Geometry check sheet. Reference: drawing and pictorial views, mm from the part's lowest x, y, z. A direction names the side the tool comes from. Round coordinates to 2 decimals unless told otherwise and drop trailing zeros. Write each loop counter-clockwise with the first axis right and the second up, starting at its lowest first coordinate (ties: lowest second). Pieces come first, ordered by that corner, then holes. Notation, with made-up numbers: M 62,12 L 66,12 A8 cw 66,24 Z; hole C 50.25,26 d10. An arc over 180 degrees is marked long. Answer in a Markdown table with one row per item. Add a question column.
1. Sectioned sample at D-D on z = 2. Record the cut outline in (x, y).
2. Sectioned sample at C-C on y = 21.5. Record the cut outline in (x, z), plus the area to 3 significant figures.
3. Set-up check for the marked faces 1 and 2: record each of +Z, -Z, +X, -X, +Y, -Y from which the full face is reachable in a straight line by a thin tool's end or side.
4. Go/stop test with flat-tipped pins: pin 1 Ø4 at (x, y) = (7.5, 5) entering from +Z; pin 2 Ø6 at (y, z) = (12, 3.5) entering from -X; pin 3 Ø2 at (y, z) = (22, 5.5) entering from +X. Record where each tip stops, or that it passes through.
5. Material ranges on probe 1 along Y at (x, z) = (9.25, 4); probe 2 along Z at (x, y) = (8.25, 16); probe 3 along X at (y, z) = (12.5, 7.25), recorded low to high.
6. Sectioned sample at A-A on x = 6. Record the cut outline in (y, z).
7. Sectioned sample at B-B on z = 6. Record the cut outline in (x, y), plus the area to 3 significant figures.
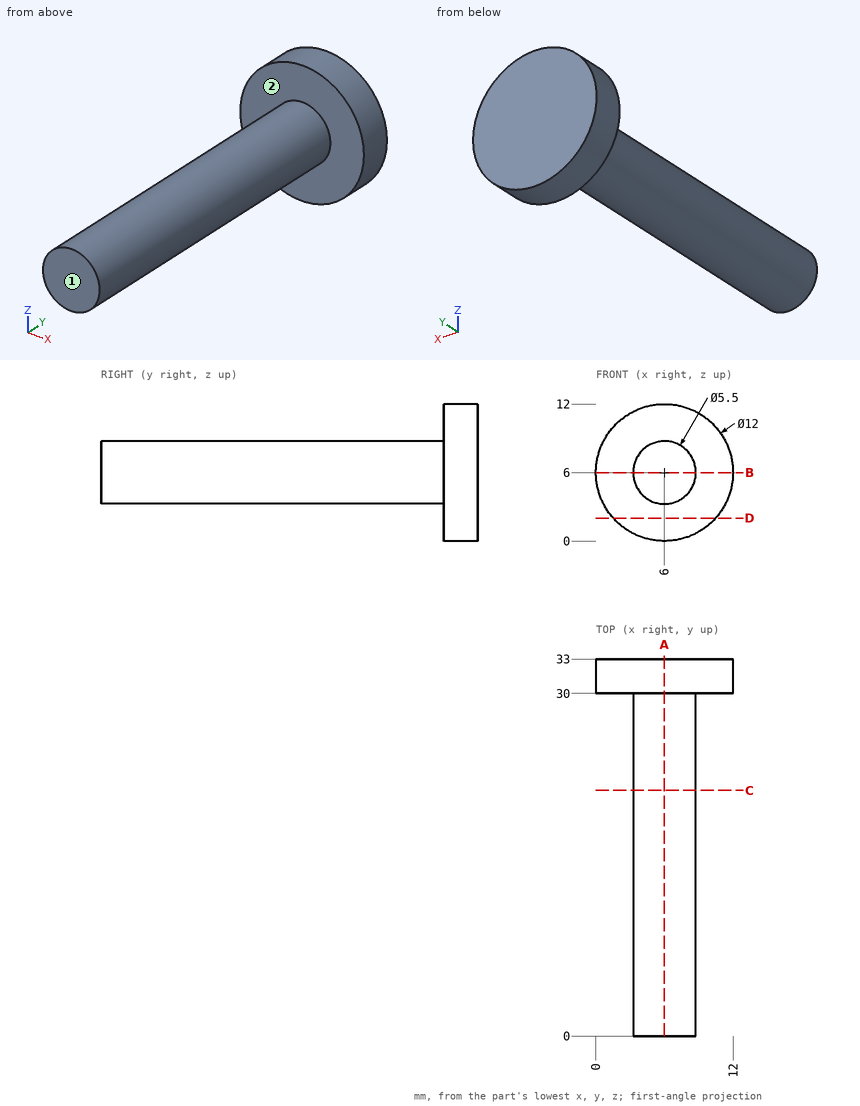
Geometry check:
| question | item | result |
|---|---|---|
| 1 | outline | M 1.53,30 L 10.47,30 L 10.47,33 L 1.53,33 Z |
| 2 | outline | C 6,6 d5.5 |
| 2 | area | 23.8 mm2 |
| 3 | face 1 | +Z, -Z, +X, -X, -Y |
| 3 | face 2 | -Y |
| 4 | pin 1 | stops at z = 8.75 |
| 4 | pin 2 | stops at x = 3.25 |
| 4 | pin 3 | stops at x = 8.75 |
| 5 | probe 1 | y = 30 to 33 |
| 5 | probe 2 | z = 4.42 to 7.58 |
| 5 | probe 3 | x = 3.55 to 8.45 |
| 6 | outline | M 0,3.25 L 30,3.25 L 30,0 L 33,0 L 33,12 L 30,12 L 30,8.75 L 0,8.75 Z |
| 7 | outline | M 0,30 L 3.25,30 L 3.25,0 L 8.75,0 L 8.75,30 L 12,30 L 12,33 L 0,33 Z |
| 7 | area | 201 mm2 |
